```python
from build123d import *

# Parameters (mm, degrees)
SKETCH1_R                      = 4
BOSS_EXTRUDE1_DEPTH            = 15
CHAMFER1_SIZE                  = 8
SKETCH2_W                      = 8
SKETCH2_H                      = 3
BOSS_EXTRUDE2_DEPTH            = 7
CHAMFER3_SIZE                  = 3
SKETCH4_W                      = 32
SKETCH4_H                      = 3
CUT_EXTRUDE2_DEPTH             = 7
CUT_EXTRUDE2_DIRECTION_2_REACH = 25.345
CUT_EXTRUDE3_REACH             = 33.559
SKETCH6_R                      = 1.75
CUT_EXTRUDE4_DEPTH             = 32.559467676
SKETCH7_W                      = 16
SKETCH7_H                      = 3
BOSS_EXTRUDE3_DEPTH            = 7


with BuildPart() as part:
    # Sketch1 → Boss-Extrude1 (new body)
    with BuildSketch(Plane(origin=(0, 0, 0), x_dir=(1, 0, 0), z_dir=(0, 1, 0))):
        Polygon((-8, -5), (-8, 5), (-16, 5), (-16, 8), (16, 8), (16, 5), (8, 5), (8, -5), (16, -5), (16, -8), (-16, -8), (-16, -5), align=None)
        with Locations(Location((0, 0, 0), (0, 0, 270))):
            Circle(SKETCH1_R, mode=Mode.SUBTRACT)
    extrude(amount=BOSS_EXTRUDE1_DEPTH)

    # Chamfer1
    chamfer1_edges = [part.edges().sort_by_distance(p)[0] for p in [
        (16, 0, 6.5),
        (-16, 0, 6.5),
        (-16, 0, -6.5),
        (16, 0, -6.5),
    ]]
    chamfer(chamfer1_edges, length=CHAMFER1_SIZE)

    # Sketch2 → Boss-Extrude2 (add)
    with BuildSketch(Plane(origin=(0, 15, 0), x_dir=(1, 0, 0), z_dir=(0, 1, 0))):
        with Locations((12, -6.5)):
            Rectangle(SKETCH2_W, SKETCH2_H)
        with Locations((12, 6.5)):
            Rectangle(SKETCH2_W, SKETCH2_H)
        with Locations((-12, -6.5)):
            Rectangle(SKETCH2_W, SKETCH2_H)
        with Locations((-12, 6.5)):
            Rectangle(SKETCH2_W, SKETCH2_H)
    extrude(amount=BOSS_EXTRUDE2_DEPTH)

    # Chamfer3
    chamfer3_edges = [part.edges().sort_by_distance(p)[0] for p in [
        (-12, 22, 8),
        (12, 22, 8),
        (-12, 22, -8),
        (12, 22, -8),
    ]]
    chamfer(chamfer3_edges, length=CHAMFER3_SIZE - 0.0001)  # a hair under: the kernel refuses the full size

    # Sketch4 → Cut-Extrude2 (cut)
    with BuildSketch(Plane(origin=(0, 15, 0), x_dir=(1, 0, 0), z_dir=(0, 1, 0))):
        with Locations((0, 6.5)):
            Rectangle(SKETCH4_W, SKETCH4_H)
    extrude(amount=-CUT_EXTRUDE2_DEPTH, mode=Mode.SUBTRACT)

    # Sketch4 → Cut-Extrude2 direction 2 (cut, up to next)
    with BuildSketch(Plane(origin=(0, 15, 0), x_dir=(1, 0, 0), z_dir=(0, 1, 0)), mode=Mode.PRIVATE) as cut_extrude2_direction_2_sk1:
        with Locations((0, 6.5)):
            Rectangle(SKETCH4_W, SKETCH4_H)
    cut_extrude2_direction_2_tool1 = extrude(cut_extrude2_direction_2_sk1.sketch, amount=CUT_EXTRUDE2_DIRECTION_2_REACH, mode=Mode.PRIVATE) & part.part
    add(cut_extrude2_direction_2_tool1.solids().sort_by_distance((0, 15, -6.5))[0], mode=Mode.SUBTRACT)


with BuildPart() as cut_extrude2_kept_piece:
    # of the separate pieces the step leaves, the one the design keeps (cut_extrude2_pieces_kept)
    add(part.part.solids().sort_by_distance((-16, 8, -5))[0])

    # Sketch5 → Cut-Extrude3 (cut, up to next)
    with BuildSketch(Plane(origin=(0, 0, -8), x_dir=(-1, 0, 0), z_dir=(0, 0, -1)), mode=Mode.PRIVATE) as cut_extrude3_sk1:
        Polygon((-12, 4), (-12, 8), (-16, 8), align=None)
    cut_extrude3_tool1 = extrude(cut_extrude3_sk1.sketch, amount=-CUT_EXTRUDE3_REACH, mode=Mode.PRIVATE) & cut_extrude2_kept_piece.part
    # Sketch5 → Cut-Extrude3 (cut, up to next)
    with BuildSketch(Plane(origin=(0, 0, -8), x_dir=(-1, 0, 0), z_dir=(0, 0, -1)), mode=Mode.PRIVATE) as cut_extrude3_sk2:
        Polygon((16, 8), (12, 4), (12, 8), align=None)
    cut_extrude3_tool2 = extrude(cut_extrude3_sk2.sketch, amount=-CUT_EXTRUDE3_REACH, mode=Mode.PRIVATE) & cut_extrude2_kept_piece.part
    add(cut_extrude3_tool1.solids().sort_by_distance((13.333333, 6.666667, -8))[0], mode=Mode.SUBTRACT)
    add(cut_extrude3_tool2.solids().sort_by_distance((-13.333333, 6.666667, -8))[0], mode=Mode.SUBTRACT)

    # Sketch6 → Cut-Extrude4 (cut, through all)
    with BuildSketch(Plane.XY.offset(8)):
        with Locations((12, 12)):
            Circle(SKETCH6_R)
        with Locations((-12, 12)):
            Circle(SKETCH6_R)
    extrude(amount=-CUT_EXTRUDE4_DEPTH, mode=Mode.SUBTRACT)

    # Sketch7 → Boss-Extrude3 (add)
    with BuildSketch(Plane(origin=(0, 8, 0), x_dir=(1, 0, 0), z_dir=(0, 1, 0))):
        with Locations((0, 6.5)):
            Rectangle(SKETCH7_W, SKETCH7_H)
    extrude(amount=BOSS_EXTRUDE3_DEPTH)


solid = cut_extrude2_kept_piece.part
```
Input: part model. Units: mm. Frame: model coordinates. A direction names the side the tool comes from. Give positions to 0.01 mm unless a question says otherwise; leave off trailing zeros. Loops run counter-clockwise (first coordinate to the right, second up) from the corner with the lowest first, then second, coordinate; pieces in that order, holes last.
1) Section query A-A on y = 12. Return the cut outline in (x, z), and give its area (3 significant figures).
A:
outline: (-16, 5) - (-13.75, 5) - (-13.75, 8) - (-16, 8) - close; (-10.25, 5) - (-8, 5) - (-8, -8) - (8, -8) - (8, 5) - (10.25, 5) - (10.25, 8) - (-10.25, 8) - close; (13.75, 5) - (16, 5) - (16, 8) - (13.75, 8) - close; hole circle Ø8 at (0, 0)
area: 233 mm2
2) Mould query, pull axis X, two halves, no side actions, for faces 1 (the flat face through (10, 2, -7)), 2 (the flat face through (-12, 20, 7)), 3 (the flat face through (-16, 15, 7)), 4 (the cylindrical face through (-3.905, 7.395, -0.867)). Classes: released by +X, released by -X, zero draft, split by the parting line, or undercut.
A:
face 1: released by +X
face 2: zero draft
face 3: released by -X
face 4: undercut
3) Contact query for flat-ended pins moving along their axis: pin 1 (2.5 mm diameter, centred on y = 5.5, z = -6.5, fed in from +X); pin 2 (0.9 mm diameter, centred on x = 10, z = -6.5, fed in from +Y); pin 3 (1.5 mm diameter, centred on y = 6.5, z = -7, fed in from -X). Output: stop coordinate, or through.
A:
pin 1: stops at x = 12
pin 2: stops at y = 8
pin 3: stops at x = -12
4) Line query: L1, parallel to Z at x = -11.5, y = 7.5; L2, parallel to X at y = 18, z = 5.5; L3, parallel to Z at x = 11, y = 19. Output: solid intervals per line, ascending.
A:
L1: z = -8 to -5, 5 to 8
L2: x = -16 to -8, 8 to 16
L3: z = 5 to 8
5) Section query D-D on z = -5.75. Return the cut outline in (x, y), and give its area (3 significant figures).
A:
outline: (-12, 4) - (-8, 0) - (8, 0) - (12, 4) - (12, 8) - (8, 8) - (8, 15) - (-8, 15) - (-8, 8) - (-12, 8) - close
area: 288 mm2
6) Section query C-C on y = 18.5. Return the cut outline in (x, z).
A:
outline: (-16, 5) - (-8, 5) - (-8, 8) - (-16, 8) - close; (8, 5) - (16, 5) - (16, 8) - (8, 8) - close
7) Reachability of faces 5 (the flat face through (10, 8, -7)), 6 (the flat face through (-10, 8, -7)), 7 (the flat face through (-10, 5, -5)), 8 (the flat face through (-4, 15, -2)) from +Z, -Z, +X, -X, +Y, -Y: full face, straight path, thin tool, end or side. Return the list, or none.
A:
face 5: -Z, +X, +Y
face 6: -Z, -X, +Y
face 7: -X, +Y, -Y
face 8: +Z, -Z, +Y
8) Section query B-B on x = 0. Return the cut outline in (y, z), and give its area (3 significant figures).
A:
outline: (0, -8) - (15, -8) - (15, -4) - (0, -4) - close; (0, 4) - (15, 4) - (15, 8) - (0, 8) - close
area: 120 mm2
